Geometry check sheet. Reference: the model listing, model coordinates, mm. Round coordinates to 2 decimals unless told otherwise and drop trailing zeros. Order: outer loops, then holes, each group sorted by start corner. A loop starts at its lowest first (then second) coordinate and runs counter-clockwise, first axis right, second up.
(1) Gauge pin test, flat ends, axial feed: P1, Ø5.5, axis at x = -159.42, y = -44.07, coming from the -Z side; P2, Ø1.5, axis at x = 85, z = 5, coming from the +Y side; P3, Ø1, axis at x = -140, z = 6, coming from the -Y side; P4, Ø2, axis at x = 107, z = 6, coming from the +Y side. Record the tip position at first contact, or that the pin passes through.
(2) Thickness scan on L1, parallel to Y at x = 126.5, z = 8.75; L2, parallel to Y at x = 16.5, z = 4; L3, parallel to X at y = 160.1, z = 2.75. Record the ranges inside material, lowest first.
(3) Draft check along Y on faces 1 (the face through (-3, 3, 9)), 2 (the face through (174.94, -99.36, 4.44)), 3 (the face through (-135, 0, 4)). Enter one of: pulls with the +Y half, pulls with the -Y half, needs draft (parallel to the pull), parting line crosses it, or undercut.
(4) Cross-section at B-B on y = -148.1. Enter the section's corners in (x, z).
(5) Cross-section at D-D on x = -149. Enter the section's corners in (y, z), and give its area (3 significant figures).
(6) Cross-section at C-C on x = -21.5. Enter the section's corners in (y, z).
(7) Cross-section at A-A on y = 74.05. Enter the section's corners in (x, z).
Autodesk Inventor part; units mm, degrees
ref_plane "YZ Plane" through (0, 0, 0) normal (1, 0, 0) x (0, 1, 0)
ref_plane "XZ Plane" through (0, 0, 0) normal (0, 1, 0) x (-1, 0, 0)
ref_plane "XY Plane" through (0, 0, 0) normal (0, 0, 1) x (1, 0, 0)
sketch "Sketch1" plane through (0, 0, 0) normal (0, 0, 1) x (1, 0, 0)
  circle A0 centre (0, 0) radius 186.2 construction
  line L0 (0, 0) -> (0, 152.9684) construction
  circle A1 centre (0, 0) radius 100 construction
  circle A2 centre (0, 148.1) radius 38.1
  circle A3 centre (0, 148.1) radius 37.5 construction
  arc A4 (-52.8521, 124.2242) -> (-81.1553, 107.8834) centre (0, 0) ccw
  arc A5 (-134.0074, 16.3409) -> (-134.0074, -16.3409) centre (0, 0) ccw
  arc A6 (-81.1553, -107.8834) -> (-52.8521, -124.2242) centre (0, 0) ccw
  arc A7 (52.8521, -124.2242) -> (81.1553, -107.8834) centre (0, 0) ccw
  arc A8 (134.0074, -16.3409) -> (134.0074, 16.3409) centre (0, 0) ccw
  arc A9 (81.1553, 107.8834) -> (52.8521, 124.2242) centre (0, 0) ccw
  arc A10 (50.0927, 130.4839) -> (-50.0927, 130.4839) centre (0, 148.1) ccw
  arc A11 (-52.8521, 124.2242) -> (-50.0927, 130.4839) centre (-54.8096, 128.8251) ccw
  arc A12 (50.0927, 130.4839) -> (52.8521, 124.2242) centre (54.8096, 128.8251) ccw
  arc A13 (-87.956, 108.6235) -> (-138.0487, 21.8604) centre (-128.2584, 74.05) ccw
  circle A14 centre (-128.2584, 74.05) radius 38.1
  arc A15 (-87.956, 108.6235) -> (-81.1553, 107.8834) centre (-84.161, 111.879) ccw
  arc A16 (-134.0074, 16.3409) -> (-138.0487, 21.8604) centre (-138.9706, 16.9461) ccw
  arc A17 (-138.0487, -21.8604) -> (-87.956, -108.6235) centre (-128.2584, -74.05) ccw
  circle A18 centre (-128.2584, -74.05) radius 38.1
  arc A19 (-138.0487, -21.8604) -> (-134.0074, -16.3409) centre (-138.9706, -16.9461) ccw
  arc A20 (-81.1553, -107.8834) -> (-87.956, -108.6235) centre (-84.161, -111.879) ccw
  arc A21 (-50.0927, -130.4839) -> (50.0927, -130.4839) centre (0, -148.1) ccw
  circle A22 centre (0, -148.1) radius 38.1
  arc A23 (-50.0927, -130.4839) -> (-52.8521, -124.2242) centre (-54.8096, -128.8251) ccw
  arc A24 (52.8521, -124.2242) -> (50.0927, -130.4839) centre (54.8096, -128.8251) ccw
  arc A25 (87.956, -108.6235) -> (138.0487, -21.8604) centre (128.2584, -74.05) ccw
  circle A26 centre (128.2584, -74.05) radius 38.1
  arc A27 (87.956, -108.6235) -> (81.1553, -107.8834) centre (84.161, -111.879) ccw
  arc A28 (134.0074, -16.3409) -> (138.0487, -21.8604) centre (138.9706, -16.9461) ccw
  arc A29 (138.0487, 21.8604) -> (87.956, 108.6235) centre (128.2584, 74.05) ccw
  circle A30 centre (128.2584, 74.05) radius 38.1
  arc A31 (138.0487, 21.8604) -> (134.0074, 16.3409) centre (138.9706, 16.9461) ccw
  arc A32 (81.1553, 107.8834) -> (87.956, 108.6235) centre (84.161, 111.879) ccw
  circle A33 centre (41.5415, 160.1) radius 3.3
  circle A34 centre (41.5415, 136.1) radius 3.3
  line L1 (0, 148.1) -> (41.5415, 160.1) construction
  line L2 (41.5415, 160.1) -> (41.5415, 136.1) construction
  line L3 (41.5415, 136.1) -> (0, 148.1) construction
  circle A35 centre (-41.5415, 160.1) radius 3.3
  circle A36 centre (-41.5415, 136.1) radius 3.3
  circle A37 centre (-117.8799, 116.026) radius 3.3
  circle A38 centre (-97.0953, 104.026) radius 3.3
  circle A39 centre (-159.4214, 44.074) radius 3.3
  circle A40 centre (-138.6368, 32.074) radius 3.3
  circle A41 centre (-159.4214, -44.074) radius 3.3
  circle A42 centre (-138.6368, -32.074) radius 3.3
  circle A43 centre (-117.8799, -116.026) radius 3.3
  circle A44 centre (-97.0953, -104.026) radius 3.3
  circle A45 centre (-41.5415, -160.1) radius 3.3
  circle A46 centre (-41.5415, -136.1) radius 3.3
  circle A47 centre (41.5415, -160.1) radius 3.3
  circle A48 centre (41.5415, -136.1) radius 3.3
  circle A49 centre (117.8799, -116.026) radius 3.3
  circle A50 centre (97.0953, -104.026) radius 3.3
  circle A51 centre (159.4214, -44.074) radius 3.3
  circle A52 centre (138.6368, -32.074) radius 3.3
  circle A53 centre (159.4214, 44.074) radius 3.3
  circle A54 centre (138.6368, 32.074) radius 3.3
  circle A55 centre (117.8799, 116.026) radius 3.3
  circle A56 centre (97.0953, 104.026) radius 3.3
  circle A57 centre (0, 0) radius 72.5 construction
  line L4 (0, 0) -> (293.3984, 0) construction
  line L5 (0, 0) -> (-240, 0) construction
  circle A58 centre (0, 40) radius 3.9
  circle A59 centre (-34.641, 20) radius 3.9
  circle A60 centre (-34.641, -20) radius 3.9
  circle A61 centre (0, -40) radius 3.9
  circle A62 centre (34.641, -20) radius 3.9
  circle A63 centre (34.641, 20) radius 3.9
  circle A64 centre (-120, 0) radius 3.9
  circle A65 centre (-60, -103.923) radius 3.9
  circle A66 centre (60, -103.923) radius 3.9
  circle A67 centre (120, 0) radius 3.9
  circle A68 centre (60, 103.923) radius 3.9
  circle A69 centre (-60, 103.923) radius 3.9
  point P0 (-34.3824, 131.6848)
  point P1 (-32.4194, 128.0852)
  point P2 (34.2525, 131.4155)
  point P3 (32.4194, 128.0852)
  point P4 (-94.7153, 92.1186)
  point P5 (-127.1347, 35.9666)
  point P6 (-131.2335, 36.0663)
  point P7 (-96.6829, 95.3713)
  point P8 (-127.1347, -35.9666)
  point P9 (-94.7153, -92.1186)
  point P10 (-96.8511, -95.6184)
  point P11 (-130.9354, -36.0442)
  point P12 (-32.4194, -128.0852)
  point P13 (32.4194, -128.0852)
  point P14 (34.3824, -131.6848)
  point P15 (-34.2525, -131.4155)
  point P16 (94.7153, -92.1186)
  point P17 (127.1347, -35.9666)
  point P18 (131.2335, -36.0663)
  point P19 (96.6829, -95.3713)
  point P20 (127.1347, 35.9666)
  point P21 (94.7153, 92.1186)
  point P22 (96.8511, 95.6184)
  point P23 (130.9354, 36.0442)
  dimension "d0" = 372.4
  dimension "d42" = 0.6
  dimension "d43" = 135
  dimension "d44" = 75
  dimension "d45" = 15
  dimension "d48" = 5
  dimension "d51" = 360
  dimension "d53" = 6.6
  dimension "d54" = 6.6
  dimension "d56" = 43.24
  dimension "d57" = 24
  dimension "d58" = 43.24
  dimension "d61" = 360
  dimension "d64" = 200
  dimension "d65" = 145
  dimension "d73" = 7.8
  dimension "d74" = 40
  dimension "d77" = 360
  dimension "d79" = 7.8
  dimension "d80" = 120
  dimension "d83" = 360
extrude "Extrusion1" add sketch "Sketch1" along normal blind 9
properties part number "GenevaHolder" material "Plywood, Finish"
Found:
1. P1: passes through
1. P2: stops at y = 107.14
1. P3: stops at y = -125.95
1. P4: stops at y = 123.13
2. L1: y = -127.12 to -112.11, -35.99 to 35.99, 112.11 to 127.12
2. L2: y = -198.57 to -182.44, -113.76 to 113.76, 182.44 to 198.57
2. L3: x = -51.73 to -44.84, -38.24 to -36.16, 36.16 to 38.24, 44.84 to 51.73
3. face 1: needs draft
3. face 2: undercut
3. face 3: undercut
4. outline: (-53.1, 0) - (-38.1, 0) - (-38.1, 9) - (-53.1, 9) - close; (38.1, 0) - (53.1, 0) - (53.1, 9) - (38.1, 9) - close
5. outline: (-122.93, 0) - (-106.01, 0) - (-106.01, 9) - (-122.93, 9) - close; (-42.09, 0) - (-25.17, 0) - (-25.17, 9) - (-42.09, 9) - close; (25.17, 0) - (42.09, 0) - (42.09, 9) - (25.17, 9) - close; (106.01, 0) - (122.93, 0) - (122.93, 9) - (106.01, 9) - close
5. area: 609 mm2
6. outline: (-196.65, 0) - (-179.55, 0) - (-179.55, 9) - (-196.65, 9) - close; (-116.65, 0) - (116.65, 0) - (116.65, 9) - (-116.65, 9) - close; (179.55, 0) - (196.65, 0) - (196.65, 9) - (179.55, 9) - close
7. outline: (-181.36, 0) - (-166.36, 0) - (-166.36, 9) - (-181.36, 9) - close; (-90.16, 0) - (90.16, 0) - (90.16, 9) - (-90.16, 9) - close; (166.36, 0) - (181.36, 0) - (181.36, 9) - (166.36, 9) - close
